Autodesk Inventor part; units mm, degrees
ref_plane "YZ Plane" through (0, 0, 0) normal (1, 0, 0) x (0, 1, 0)
ref_plane "XZ Plane" through (0, 0, 0) normal (0, 1, 0) x (-1, 0, 0)
ref_plane "XY Plane" through (0, 0, 0) normal (0, 0, 1) x (1, 0, 0)
sketch "Sketch1" plane through (0, 0, 0) normal (0, 0, 1) x (1, 0, 0)
  line L0 (11, 50) -> (11, 0)
  line L1 (11, 0) -> (16, 0)
  line L2 (16, 0) -> (16, 2.88)
  line L3 (11, 50) -> (0, 50)
  line L4 (0, 50) -> (0, 100) construction
  line L5 (11, 100) -> (16, 100)
  line L6 (16, 100) -> (16, 2.88)
  circle A0 centre (13.5, 7.75) radius 1.25
  circle A1 centre (13.5, 15.75) radius 1.25
  circle A2 centre (13.5, 23.75) radius 1.25
  circle A3 centre (13.5, 31.75) radius 1.25
  line L7 (-11, 50) -> (-11, 0)
  line L8 (-11, 0) -> (-16, 0)
  line L9 (-11, 50) -> (0, 50)
  line L10 (-11, 100) -> (-16, 100)
  line L11 (-16, 100) -> (-16, 2.88)
  circle A4 centre (-13.5, 7.75) radius 1.25
  circle A5 centre (-13.5, 15.75) radius 1.25
  circle A6 centre (-13.5, 23.75) radius 1.25
  circle A7 centre (-13.5, 31.75) radius 1.25
  line L12 (-16, 2.88) -> (-16, 0)
  line L13 (-11, 100) -> (-11, 75)
  line L14 (-11, 75) -> (11, 75)
  line L15 (11, 75) -> (11, 100)
  point P0 (0, 0)
  dimension "d0" = 5
  dimension "d1" = 100
  dimension "d2" = 11
  dimension "d3" = 50
  dimension "d4" = 0
  dimension "d5" = 0
  dimension "d6" = 2.5
  dimension "d7" = 2.5
  dimension "d8" = 7.75
  dimension "d9" = 0
  dimension "d10" = 8
  dimension "d11" = 2.5
  dimension "d12" = 0
  dimension "d13" = 8
  dimension "d14" = 2.5
  dimension "d15" = 2.5
  dimension "d16" = 0
  dimension "d17" = 8
  dimension "d18" = 5
  dimension "d19" = 5
  dimension "d20" = 25
  dimension "d21" = 0
extrude "Extrusion1" add sketch "Sketch1" along normal blind 5
equation "\"d11\" = d6"
equation "\"d14\" = d6"
equation "\"d15\" = d6"
properties part number "Bridge"
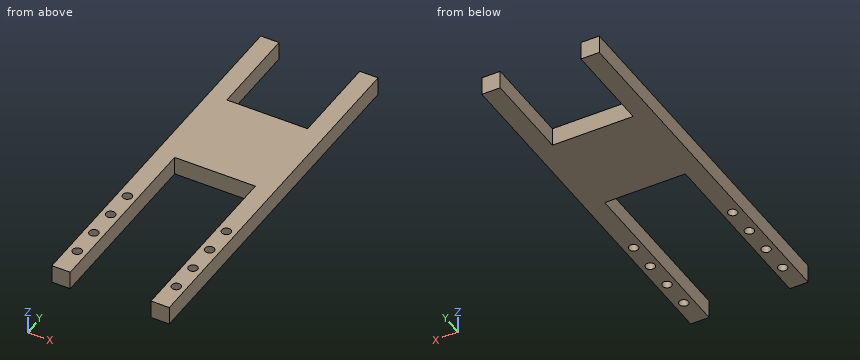
Part model, mm, in its own coordinate system. Give positions to 0.01 mm unless a question says otherwise; leave off trailing zeros. Order: outer loops, then holes, each group sorted by start corner. A loop starts at its lowest first (then second) coordinate and runs counter-clockwise, first axis right, second up. Notation, with made-up numbers: (47.5, 37.5) - (103.5, 37.5) arc R20 ccw to (103.5, 61.5) - close; hole circle Ø8 at (54, -9). An arc over 180 degrees is marked (long way). Use a Markdown table: item, result.
1) Saw through at A-A on x = -13.5. List the corners of the cut face in (y, z).
Checked values:
| item | result |
|---|---|
| outline | (0, 0) - (6.5, 0) - (6.5, 5) - (0, 5) - close; (9, 0) - (14.5, 0) - (14.5, 5) - (9, 5) - close; (17, 0) - (22.5, 0) - (22.5, 5) - (17, 5) - close; (25, 0) - (30.5, 0) - (30.5, 5) - (25, 5) - close; (33, 0) - (100, 0) - (100, 5) - (33, 5) - close |
2) Flat gauge pins, fed straight in: P1, Ø4, axis at x = -2.5, y = 77.5, coming from the +Z side; P2, Ø2.5, axis at x = 4.5, z = 2, coming from the +Y side. Where does each tip first touch, or does it go through?
Checked values:
| item | result |
|---|---|
| P1 | through |
| P2 | y = 75 |
3) Saw through at D-D on y = 31.75. List the corners of the cut face in (x, z), plus the area to 3 significant figures.
Checked values:
| item | result |
|---|---|
| outline | (-16, 0) - (-14.75, 0) - (-14.75, 5) - (-16, 5) - close; (-12.25, 0) - (-11, 0) - (-11, 5) - (-12.25, 5) - close; (11, 0) - (12.25, 0) - (12.25, 5) - (11, 5) - close; (14.75, 0) - (16, 0) - (16, 5) - (14.75, 5) - close |
| area | 25.0 mm² |
4) Saw through at C-C on z = 2.7. Count the separate pieces of the cut face and the enclosed holes in it, plus the area to 3 significant figures.
Checked values:
| item | result |
|---|---|
| separate pieces | 1 |
| enclosed holes | 8 |
| area | 1,510 mm² |
5) Saw through at B-B on y = 77. List the corners of the cut face in (x, z).
Checked values:
| item | result |
|---|---|
| outline | (-16, 0) - (-11, 0) - (-11, 5) - (-16, 5) - close; (11, 0) - (16, 0) - (16, 5) - (11, 5) - close |
6) Probe L1, parallel to Y at x = 13.5, z = 2.4; L2, parallel to X at y = 42.5, z = 2.6; L3, parallel to Y at x = 14, z = 0.85. List the from-to ranges inside material, lowest first. Write a range as from..to.
Checked values:
| item | result |
|---|---|
| L1 | 0..6.5, 9..14.5, 17..22.5, 25..30.5, 33..100 |
| L2 | -16..-11, 11..16 |
| L3 | 0..6.6, 8.9..14.6, 16.9..22.6, 24.9..30.6, 32.9..100 |
